```python
from build123d import *

# Parameters (mm, degrees)
F0_R     = 4.58
F0_R_2   = 8
F1_DEPTH = 3


with BuildPart() as f1:
    # F0 (on Top) → F1 (new body)
    with BuildSketch(Plane.XY):
        with BuildLine():
            ThreePointArc((6.614378, 27.5), (0, 45), (-6.614378, 27.5))
            ThreePointArc((-6.614378, 27.5), (-8.379534, 25.457418), (-9.533996, 23.017103))
            ThreePointArc((-9.533996, 23.017103), (-12.075887, 23.926338), (-14.768365, 24.122508))
            ThreePointArc((-14.768365, 24.122508), (-31.819805, 31.819805), (-24.122508, 14.768365))
            ThreePointArc((-24.122508, 14.768365), (-23.926338, 12.075887), (-23.017103, 9.533996))
            ThreePointArc((-23.017103, 9.533996), (-25.457418, 8.379534), (-27.5, 6.614378))
            ThreePointArc((-27.5, 6.614378), (-45, 0), (-27.5, -6.614378))
            ThreePointArc((-27.5, -6.614378), (-25.457418, -8.379534), (-23.017103, -9.533996))
            ThreePointArc((-23.017103, -9.533996), (-23.926338, -12.075887), (-24.122508, -14.768365))
            ThreePointArc((-24.122508, -14.768365), (-31.819805, -31.819805), (-14.768365, -24.122508))
            ThreePointArc((-14.768365, -24.122508), (-12.075887, -23.926338), (-9.533996, -23.017103))
            ThreePointArc((-9.533996, -23.017103), (-8.379534, -25.457418), (-6.614378, -27.5))
            ThreePointArc((-6.614378, -27.5), (0, -45), (6.614378, -27.5))
            ThreePointArc((6.614378, -27.5), (8.379534, -25.457418), (9.533996, -23.017103))
            ThreePointArc((9.533996, -23.017103), (12.075887, -23.926338), (14.768365, -24.122508))
            ThreePointArc((14.768365, -24.122508), (31.819805, -31.819805), (24.122508, -14.768365))
            ThreePointArc((24.122508, -14.768365), (23.926338, -12.075887), (23.017103, -9.533996))
            ThreePointArc((23.017103, -9.533996), (25.457418, -8.379534), (27.5, -6.614378))
            ThreePointArc((27.5, -6.614378), (45, 0), (27.5, 6.614378))
            ThreePointArc((27.5, 6.614378), (25.457418, 8.379534), (23.017103, 9.533996))
            ThreePointArc((23.017103, 9.533996), (23.926338, 12.075887), (24.122508, 14.768365))
            ThreePointArc((24.122508, 14.768365), (31.819805, 31.819805), (14.768365, 24.122508))
            ThreePointArc((14.768365, 24.122508), (12.075887, 23.926338), (9.533996, 23.017103))
            ThreePointArc((9.533996, 23.017103), (8.379534, 25.457418), (6.614378, 27.5))
        make_face()
        with Locations((-24.748737, -24.748737)):
            Circle(F0_R, mode=Mode.SUBTRACT)
        with Locations((-14.142136, -14.142136)):
            Circle(F0_R, mode=Mode.SUBTRACT)
        with Locations((0, -35)):
            Circle(F0_R, mode=Mode.SUBTRACT)
        with Locations((24.748737, -24.748737)):
            Circle(F0_R, mode=Mode.SUBTRACT)
        with Locations((0, -20)):
            Circle(F0_R, mode=Mode.SUBTRACT)
        with Locations((14.142136, -14.142136)):
            Circle(F0_R, mode=Mode.SUBTRACT)
        with Locations((-35, 0)):
            Circle(F0_R, mode=Mode.SUBTRACT)
        with Locations((-20, 0)):
            Circle(F0_R, mode=Mode.SUBTRACT)
        with Locations((-14.142136, 14.142136)):
            Circle(F0_R, mode=Mode.SUBTRACT)
        with Locations((-24.748737, 24.748737)):
            Circle(F0_R, mode=Mode.SUBTRACT)
        Circle(F0_R_2, mode=Mode.SUBTRACT)
        with Locations((20, 0)):
            Circle(F0_R, mode=Mode.SUBTRACT)
        with Locations((0, 20)):
            Circle(F0_R, mode=Mode.SUBTRACT)
        with Locations((14.142136, 14.142136)):
            Circle(F0_R, mode=Mode.SUBTRACT)
        with Locations((35, 0)):
            Circle(F0_R, mode=Mode.SUBTRACT)
        with Locations((0, 35)):
            Circle(F0_R, mode=Mode.SUBTRACT)
        with Locations((24.748737, 24.748737)):
            Circle(F0_R, mode=Mode.SUBTRACT)
    extrude(amount=F1_DEPTH)


solid = f1.part
```
Geometry check sheet. Reference: the model listing, model coordinates, mm. Round coordinates to 2 decimals unless told otherwise and drop trailing zeros. Write each loop counter-clockwise with the first axis right and the second up, starting at its lowest first coordinate (ties: lowest second). Pieces come first, ordered by that corner, then holes. Notation, with made-up numbers: (84, 78.25) - (91, 78.25) arc R26 ccw to (91, 93.25) - close; hole circle Ø9 at (86.25, -31.5). An arc over 180 degrees is marked (long way). Write each question's results on one line, items separated by ' | '.
(1) Draft check along Y on faces 1 (the face through (-1, 11, 3)), 2 (the face through (8.4, 25.426, 1.479)). Enter one of: pulls with the +Y half, pulls with the -Y half, needs draft (parallel to the pull), parting line crosses it, or undercut.
Computed:
face 1: needs draft | face 2: undercut
(2) Thickness scan on probe 1 along Y at (x, z) = (-27.5, 2.65); probe 2 along X at (y, z) = (26.5, 2.6); probe 3 along X at (y, z) = (-17.5, 0.3). Record the ranges inside material, lowest first. Write a range as from..to.
Computed:
probe 1: y = -34.36..-28.41, -21.09..-15.13, -6.61..6.61, 15.13..21.09, 28.41..34.36 | probe 2: x = -34.59..-28.98, -20.52..-14.9, -7.6..7.6, 14.9..20.52, 28.98..34.59 | probe 3: x = -31.64..-17.26, -11.03..-3.84, 3.84..11.03, 17.26..31.64
(3) Depth check by flat-ended pin: pin 1 Ø14.5 at (x, y) = (-35, 0) entering from +Z; pin 2 Ø1 at (y, z) = (-13.5, 2.5) entering from +X; pin 3 Ø1 at (x, z) = (9, 0.5) entering from +Y. Enter the tip coordinate at first touch or a pass-through.
Computed:
pin 1: stops at z = 3 | pin 2: stops at x = 24.14 | pin 3: stops at y = 40.27
(4) Sectioned sample at B-B, the plane x = 36. Enter the section's corners in (y, z).
Computed:
outline: (-9.95, 0) - (-4.47, 0) - (-4.47, 3) - (-9.95, 3) - close; (4.47, 0) - (9.95, 0) - (9.95, 3) - (4.47, 3) - close
(5) Sectioned sample at C-C, the plane z = 0.6. Count the separate pieces of the cut face and the enclosed holes in it, plus the area to 3 significant figures.
Computed:
separate pieces: 1 | enclosed holes: 17 | area: 3,430 mm^2
(6) Sectioned sample at A-A, the plane x = 0. Enter the section's corners in (y, z).
Computed:
outline: (-45, 0) - (-39.58, 0) - (-39.58, 3) - (-45, 3) - close; (-30.42, 0) - (-24.58, 0) - (-24.58, 3) - (-30.42, 3) - close; (-15.42, 0) - (-8, 0) - (-8, 3) - (-15.42, 3) - close; (8, 0) - (15.42, 0) - (15.42, 3) - (8, 3) - close; (24.58, 0) - (30.42, 0) - (30.42, 3) - (24.58, 3) - close; (39.58, 0) - (45, 0) - (45, 3) - (39.58, 3) - close
